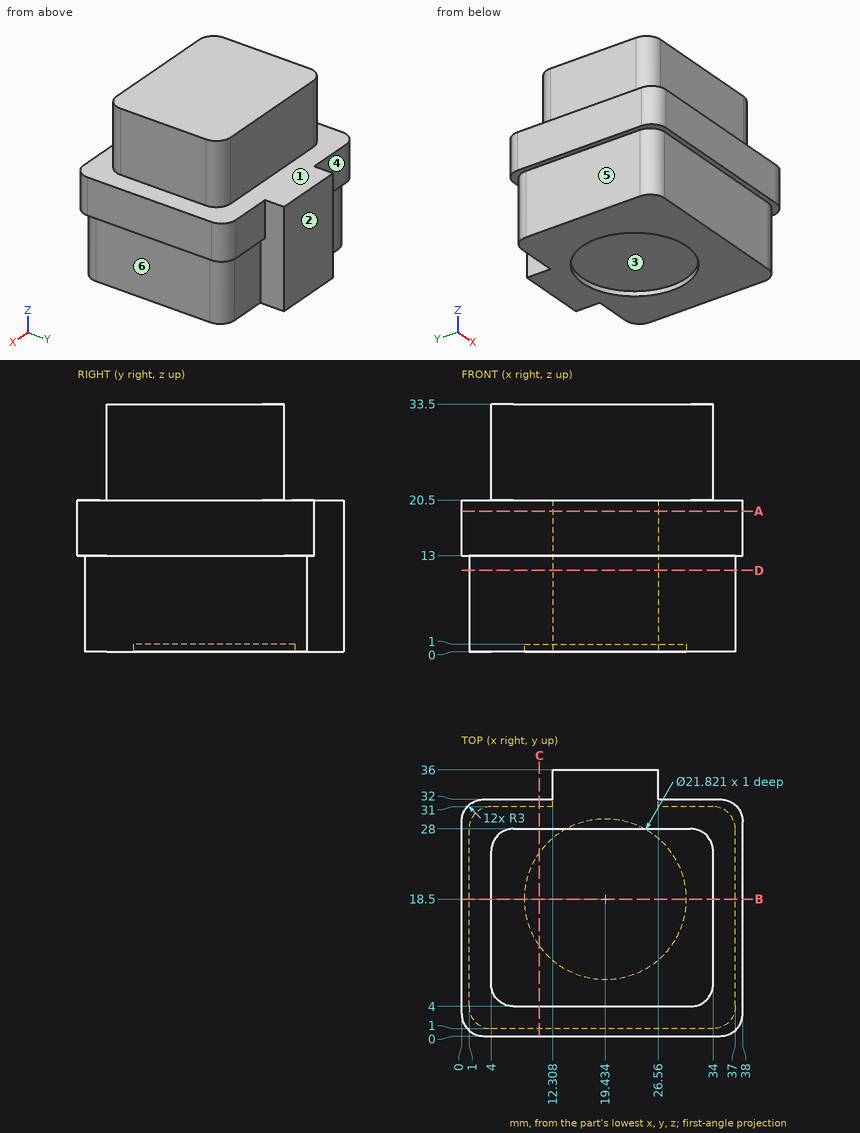
The figure shows three views and two pictorial views of one solid part (mm, origin at its lowest corner). Answer the questions. A direction names the side the tool comes from. Give positions to 0.01 mm unless a question says otherwise; leave off trailing zeros. Order: outer loops, then holes, each group sorted by start corner. A loop starts at its lowest first (then second) coordinate and runs counter-clockwise, first axis right, second up. Notation, with made-up numbers: (31.25, -1.5) -> (40.25, -1.5) arc R24 ccw to (40.25, 16.5) -> close; hole circle Ø9 at (5, 12). An arc over 180 degrees is marked (long way). Write each question's results on one line, items separated by ' | '.
Q1. Which of the six approach directions +Z, -Z, +X, -X, +Y, -Y give full straight-line access (tool end or side, diameter ignored) to the marked faces 4, 5 and 6?
Checked values:
face 4: +Z, -Z, -X, +Y | face 5: -Z, -X, +Y, -Y | face 6: -Z, +X, +Y, -Y
Q2. The part is cut by section C-C, the plane x = 10.5. Give the vertices of the cut face in (y, z).
Checked values:
outline: (0, 13) -> (1, 13) -> (1, 0) -> (12.24, 0) -> (12.24, 1) -> (24.76, 1) -> (24.76, 0) -> (31, 0) -> (31, 13) -> (32, 13) -> (32, 20.5) -> (28, 20.5) -> (28, 33.5) -> (4, 33.5) -> (4, 20.5) -> (0, 20.5) -> close
Q3. Each of these flat-tipped pins is pushed along its axis until it touches: P1, Ø2.5, axis at y = 33, z = 9.5, coming from the +X side; P2, Ø4, axis at x = 16.5, z = 5.5, coming from the -Y side; P3, Ø10.5, axis at x = 14.5, z = 26, coming from the -Y side. Where does it stop, or does it pass through?
Checked values:
P1: stops at x = 26.56 | P2: stops at y = 1 | P3: stops at y = 4
Q4. Straight lines are drawn through the part: probe 1 along X at (y, z) = (25.5, 10); probe 2 along Z at (x, y) = (19.5, 18.5); probe 3 along Z at (x, y) = (33.5, 5). For each, find the intervals that lie inside material, in ascending order. Write a range as from..to.
Checked values:
probe 1: x = 1..37 | probe 2: z = 1..33.5 | probe 3: z = 0..20.5
Q5. Determine the mould class of the marked faces 1, 2 and 3 for opening direction Y: pulls with the +Y half, pulls with the -Y half, needs draft (parallel to the pull), parting line crosses it, or undercut.
Checked values:
face 1: needs draft | face 2: pulls with the +Y half | face 3: undercut
Q6. The part is cut by section B-B, the plane y = 18.5. Give the vertices of the cut face in (x, z), and give its area (3 significant figures).
Checked values:
outline: (0, 13) -> (1, 13) -> (1, 0) -> (8.52, 0) -> (8.52, 1) -> (30.34, 1) -> (30.34, 0) -> (37, 0) -> (37, 13) -> (38, 13) -> (38, 20.5) -> (34, 20.5) -> (34, 33.5) -> (4, 33.5) -> (4, 20.5) -> (0, 20.5) -> close | area: 1,120 mm^2
Q7. The part is cut by section D-D, the plane z = 11. Give the vertices of the cut face in (x, y), and give its area (3 significant figures).
Checked values:
outline: (1, 4) arc R3 ccw to (4, 1) -> (34, 1) arc R3 ccw to (37, 4) -> (37, 28) arc R3 ccw to (34, 31) -> (26.56, 31) -> (26.56, 36) -> (12.31, 36) -> (12.31, 31) -> (4, 31) arc R3 ccw to (1, 28) -> close | area: 1,140 mm^2
Q8. The part is cut by section A-A, the plane z = 19. Give the vertices of the cut face in (x, y).
Checked values:
outline: (0, 3) arc R3 ccw to (3, 0) -> (35, 0) arc R3 ccw to (38, 3) -> (38, 29) arc R3 ccw to (35, 32) -> (26.56, 32) -> (26.56, 36) -> (12.31, 36) -> (12.31, 32) -> (3, 32) arc R3 ccw to (0, 29) -> close
